Verification items for the finished model (mm, model axes). Face numbers are marked on the shaded views. A direction names the side the tool comes from. Give positions to 0.01 mm unless a question says otherwise; leave off trailing zeros. Write each loop counter-clockwise with the first axis right and the second up, starting at its lowest first coordinate (ties: lowest second). Pieces come first, ordered by that corner, then holes. Notation, with made-up numbers: (4, -33) - (19, -33) arc R10 cw to (19, -25) - close; hole circle Ø3 at (57.25, -18.75). An arc over 180 degrees is marked (long way). Put each result on its own line as item: value.
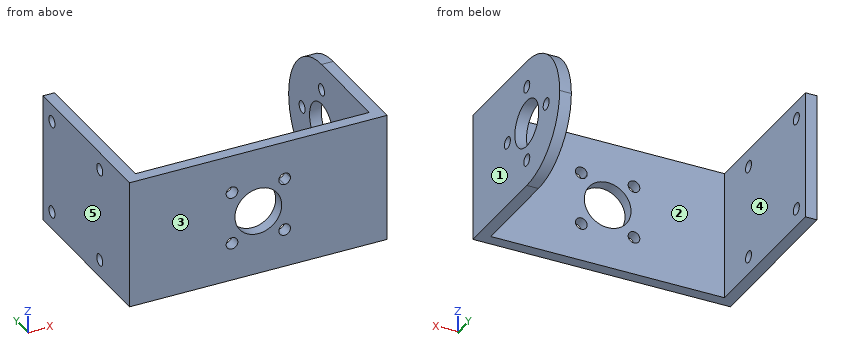
from build123d import *

# Parameters (mm, degrees)
SKETCH1_W           = 44
SKETCH1_H           = 22
BOSS_EXTRUDE1_DEPTH = 2
SKETCH2_W           = 2
SKETCH2_H           = 22
BOSS_EXTRUDE2_DEPTH = 27
CUT_EXTRUDE1_REACH  = 46
CUT_EXTRUDE2_REACH  = 46
SKETCH4_R           = 1
CUT_EXTRUDE3_REACH  = 46
SKETCH5_R           = 4
SKETCH5_R_2         = 1
SKETCH6_R           = 1
SKETCH6_R_2         = 4
CUT_EXTRUDE4_DEPTH  = 5


with BuildPart() as part:
    # Sketch1 → Boss-Extrude1 (new body)
    with BuildSketch(Plane(origin=(0, 0, 0), x_dir=(1, 0, 0), z_dir=(0, 1, 0))):
        with Locations((22, 11)):
            Rectangle(SKETCH1_W, SKETCH1_H)
    extrude(amount=BOSS_EXTRUDE1_DEPTH)

    # Sketch2 → Boss-Extrude2 (add)
    with BuildSketch(Plane(origin=(0, 2, 0), x_dir=(1, 0, 0), z_dir=(0, 1, 0))):
        with Locations((1, 11)):
            Rectangle(SKETCH2_W, SKETCH2_H)
        with Locations((43, 11)):
            Rectangle(SKETCH2_W, SKETCH2_H)
    extrude(amount=BOSS_EXTRUDE2_DEPTH)

    # Sketch3 → Cut-Extrude1 (cut, up to next)
    with BuildSketch(Plane(origin=(44, 0, 0), x_dir=(0, 0, -1), z_dir=(1, 0, 0)), mode=Mode.PRIVATE) as cut_extrude1_sk1:
        with BuildLine():
            Line((11, 29), (0, 29))
            Line((0, 29), (0, 18))
            ThreePointArc((0, 18), (3.221825407, 25.778174593), (11, 29))
        make_face()
    cut_extrude1_tool1 = extrude(cut_extrude1_sk1.sketch, amount=-CUT_EXTRUDE1_REACH, mode=Mode.PRIVATE) & part.part
    add(cut_extrude1_tool1.solids().sort_by_distance((44, 26.542953, -2.457047))[0], mode=Mode.SUBTRACT)
    # Sketch3 → Cut-Extrude1 (cut, up to next)
    with BuildSketch(Plane(origin=(44, 0, 0), x_dir=(0, 0, -1), z_dir=(1, 0, 0)), mode=Mode.PRIVATE) as cut_extrude1_sk2:
        with BuildLine():
            Line((22, 29), (11, 29))
            ThreePointArc((11, 29), (18.778174593, 25.778174593), (22, 18))
            Line((22, 18), (22, 29))
        make_face()
    cut_extrude1_tool2 = extrude(cut_extrude1_sk2.sketch, amount=-CUT_EXTRUDE1_REACH, mode=Mode.PRIVATE) & part.part
    add(cut_extrude1_tool2.solids().sort_by_distance((44, 26.542953, -19.542953))[0], mode=Mode.SUBTRACT)

    # Sketch4 → Cut-Extrude2 (cut, up to next)
    with BuildSketch(Plane.ZY, mode=Mode.PRIVATE) as cut_extrude2_sk1:
        with Locations((-19, 10)):
            Circle(SKETCH4_R)
    cut_extrude2_tool1 = extrude(cut_extrude2_sk1.sketch, amount=-CUT_EXTRUDE2_REACH, mode=Mode.PRIVATE) & part.part
    add(cut_extrude2_tool1.solids().sort_by_distance((0, 10, -19))[0], mode=Mode.SUBTRACT)
    # Sketch4 → Cut-Extrude2 (cut, up to next)
    with BuildSketch(Plane.ZY, mode=Mode.PRIVATE) as cut_extrude2_sk2:
        with Locations((-19, 26)):
            Circle(SKETCH4_R)
    cut_extrude2_tool2 = extrude(cut_extrude2_sk2.sketch, amount=-CUT_EXTRUDE2_REACH, mode=Mode.PRIVATE) & part.part
    add(cut_extrude2_tool2.solids().sort_by_distance((0, 26, -19))[0], mode=Mode.SUBTRACT)
    # Sketch4 → Cut-Extrude2 (cut, up to next)
    with BuildSketch(Plane.ZY, mode=Mode.PRIVATE) as cut_extrude2_sk3:
        with Locations((-3, 10)):
            Circle(SKETCH4_R)
    cut_extrude2_tool3 = extrude(cut_extrude2_sk3.sketch, amount=-CUT_EXTRUDE2_REACH, mode=Mode.PRIVATE) & part.part
    add(cut_extrude2_tool3.solids().sort_by_distance((0, 10, -3))[0], mode=Mode.SUBTRACT)
    # Sketch4 → Cut-Extrude2 (cut, up to next)
    with BuildSketch(Plane.ZY, mode=Mode.PRIVATE) as cut_extrude2_sk4:
        with Locations((-3, 26)):
            Circle(SKETCH4_R)
    cut_extrude2_tool4 = extrude(cut_extrude2_sk4.sketch, amount=-CUT_EXTRUDE2_REACH, mode=Mode.PRIVATE) & part.part
    add(cut_extrude2_tool4.solids().sort_by_distance((0, 26, -3))[0], mode=Mode.SUBTRACT)

    # Sketch5 → Cut-Extrude3 (cut, up to next)
    with BuildSketch(Plane(origin=(44, 0, 0), x_dir=(0, 0, -1), z_dir=(1, 0, 0)), mode=Mode.PRIVATE) as cut_extrude3_sk1:
        with Locations((11, 18)):
            Circle(SKETCH5_R)
    cut_extrude3_tool1 = extrude(cut_extrude3_sk1.sketch, amount=-CUT_EXTRUDE3_REACH, mode=Mode.PRIVATE) & part.part
    add(cut_extrude3_tool1.solids().sort_by_distance((44, 18, -11))[0], mode=Mode.SUBTRACT)
    # Sketch5 → Cut-Extrude3 (cut, up to next)
    with BuildSketch(Plane(origin=(44, 0, 0), x_dir=(0, 0, -1), z_dir=(1, 0, 0)), mode=Mode.PRIVATE) as cut_extrude3_sk2:
        with Locations((17.5, 18)):
            Circle(SKETCH5_R_2)
    cut_extrude3_tool2 = extrude(cut_extrude3_sk2.sketch, amount=-CUT_EXTRUDE3_REACH, mode=Mode.PRIVATE) & part.part
    add(cut_extrude3_tool2.solids().sort_by_distance((44, 18, -17.5))[0], mode=Mode.SUBTRACT)
    # Sketch5 → Cut-Extrude3 (cut, up to next)
    with BuildSketch(Plane(origin=(44, 0, 0), x_dir=(0, 0, -1), z_dir=(1, 0, 0)), mode=Mode.PRIVATE) as cut_extrude3_sk3:
        with Locations((11, 24.5)):
            Circle(SKETCH5_R_2)
    cut_extrude3_tool3 = extrude(cut_extrude3_sk3.sketch, amount=-CUT_EXTRUDE3_REACH, mode=Mode.PRIVATE) & part.part
    add(cut_extrude3_tool3.solids().sort_by_distance((44, 24.5, -11))[0], mode=Mode.SUBTRACT)
    # Sketch5 → Cut-Extrude3 (cut, up to next)
    with BuildSketch(Plane(origin=(44, 0, 0), x_dir=(0, 0, -1), z_dir=(1, 0, 0)), mode=Mode.PRIVATE) as cut_extrude3_sk4:
        with Locations((4.5, 18)):
            Circle(SKETCH5_R_2)
    cut_extrude3_tool4 = extrude(cut_extrude3_sk4.sketch, amount=-CUT_EXTRUDE3_REACH, mode=Mode.PRIVATE) & part.part
    add(cut_extrude3_tool4.solids().sort_by_distance((44, 18, -4.5))[0], mode=Mode.SUBTRACT)
    # Sketch5 → Cut-Extrude3 (cut, up to next)
    with BuildSketch(Plane(origin=(44, 0, 0), x_dir=(0, 0, -1), z_dir=(1, 0, 0)), mode=Mode.PRIVATE) as cut_extrude3_sk5:
        with Locations((11, 11.5)):
            Circle(SKETCH5_R_2)
    cut_extrude3_tool5 = extrude(cut_extrude3_sk5.sketch, amount=-CUT_EXTRUDE3_REACH, mode=Mode.PRIVATE) & part.part
    add(cut_extrude3_tool5.solids().sort_by_distance((44, 11.5, -11))[0], mode=Mode.SUBTRACT)

    # Sketch6 → Cut-Extrude4 (cut)
    with BuildSketch(Plane(origin=(0, 2, 0), x_dir=(1, 0, 0), z_dir=(0, 1, 0))):
        with BuildLine():
            ThreePointArc((26.5, 7.5), (25.792893219, 7.207106781), (25.5, 6.5))
            Line((25.5, 6.5), (26.5, 6.5))
            Line((26.5, 6.5), (26.5, 7.5))
        make_face()
        with BuildLine():
            Line((26.5, 6.5), (25.5, 6.5))
            ThreePointArc((25.5, 6.5), (26.5, 5.5), (27.5, 6.5))
            ThreePointArc((27.5, 6.5), (27.207106781, 7.207106781), (26.5, 7.5))
            Line((26.5, 7.5), (26.5, 6.5))
        make_face()
        with Locations((17.5, 6.5)):
            Circle(SKETCH6_R)
        with Locations((17.5, 15.5)):
            Circle(SKETCH6_R)
        with Locations((26.5, 15.5)):
            Circle(SKETCH6_R)
        with Locations((22, 11)):
            Circle(SKETCH6_R_2)
    extrude(amount=-CUT_EXTRUDE4_DEPTH, mode=Mode.SUBTRACT)


solid = part.part
Q1. Release check for a two-part mould opening along X. For the marked faces 3, 4 and 5 record: released by +X, released by -X, zero draft, split by the parting line, or undercut.
Answers follow:
face 3: zero draft
face 4: undercut
face 5: released by -X
Q2. Go/stop test with flat-tipped pins: pin 1 Ø1.6 at (y, z) = (10, -19) entering from -X; pin 2 Ø1 at (x, z) = (25, -12) entering from +Y. Record where each tip stops, or that it passes through.
Answers follow:
pin 1: stops at x = 42
pin 2: passes through
Q3. Section check D-D, the plane z = -17.5. Record the cut outline in (x, y).
Answers follow:
outline: (0, 0) - (44, 0) - (44, 17) - (42, 17) - (42, 2) - (2, 2) - (2, 29) - (0, 29) - close; (42, 19) - (44, 19) - (44, 26.87) - (42, 26.87) - close
Q4. Set-up check for the marked faces 1 and 2: record each of +Z, -Z, +X, -X, +Y, -Y from which the full face is reachable in a straight line by a thin tool's end or side.
Answers follow:
face 1: +Z, -Z, +X, +Y, -Y
face 2: +Z, -Z, +Y
Q5. Section check B-B, the plane x = 22. Record the cut outline in (y, z).
Answers follow:
outline: (0, -22) - (2, -22) - (2, -15) - (0, -15) - close; (0, -7) - (2, -7) - (2, 0) - (0, 0) - close
Q6. Scan lines: line 1 along Z through (x, y) = (17.5, 0.4); line 2 along Y through (x, z) = (42.85, -11); line 3 along X through (y, z) = (24, -14.25). Record each from-to range of solid material in increasing order.
Answers follow:
line 1: z = -22 to -16.5, -14.5 to -7.5, -5.5 to 0
line 2: y = 0 to 10.5, 12.5 to 14, 22 to 23.5, 25.5 to 29
line 3: x = 0 to 2, 42 to 44
Q7. Section check C-C, the plane y = 11.5. Record the cut outline in (x, z).
Answers follow:
outline: (0, -22) - (2, -22) - (2, 0) - (0, 0) - close; (42, -22) - (44, -22) - (44, -12) - (42, -12) - close; (42, -10) - (44, -10) - (44, 0) - (42, 0) - close
Q8. Section check A-A, the plane y = 5.5. Record the cut outline in (x, z), plus the area to 3 significant figures.
Answers follow:
outline: (0, -22) - (2, -22) - (2, 0) - (0, 0) - close; (42, -22) - (44, -22) - (44, 0) - (42, 0) - close
area: 88.0 mm2
